Autodesk Inventor part; units mm, degrees
ref_plane "YZ Plane" through (0, 0, 0) normal (1, 0, 0) x (0, 1, 0)
ref_plane "XZ Plane" through (0, 0, 0) normal (0, 1, 0) x (-1, 0, 0)
ref_plane "XY Plane" through (0, 0, 0) normal (0, 0, 1) x (1, 0, 0)
sketch "Sketch1" plane through (0, 0, 0) normal (0, 1, 0) x (-1, 0, 0)
  line L0 (0, 0) -> (762, 0)
  line L1 (762, 0) -> (762, 50.8)
  line L2 (762, 50.8) -> (0, 50.8)
  line L3 (0, 50.8) -> (0, 0)
  dimension "d0" = 762
  dimension "d1" = 50.8
extrude "Extrusion1" add sketch "Sketch1" along normal blind 3.175
sketch "Sketch2" plane through (0, 3.175, 0) normal (0, 1, 0) x (1, 0, 0)
  circle A0 centre (-381, -28.575) radius 4.7625
  line L0 (0, 0) -> (-762, 0)
  line L1 (0, -50.8) -> (0, 0)
  circle A1 centre (-114.3, -12.7) radius 4.7625
  line L2 (-762, -50.8) -> (0, -50.8)
  circle A2 centre (-647.7, -12.7) radius 4.7625
  line L3 (-647.7, 0) -> (-647.7, -50.8) construction
  line L4 (-762, -50.8) -> (0, -50.8) construction
  line L5 (-114.3, -50.8) -> (-114.3, 0) construction
  circle A3 centre (-558.8, -25.4) radius 3.3734
  line L6 (-762, 0) -> (-762, -50.8)
  circle A4 centre (-495.3, -25.4) radius 3.3734
  circle A5 centre (-203.2, -25.4) radius 3.3734
  circle A6 centre (-266.7, -25.4) radius 3.3734
  dimension "d4" = 9.525
  dimension "d5" = 28.575
  dimension "d6" = 381
  dimension "d9" = 9.525
  dimension "d10" = 38.1
  dimension "d12" = 9.525
  dimension "d13" = 38.1
  dimension "d31" = 266.7
  dimension "d32" = 266.7
  dimension "d33" = 6.7469
  dimension "d34" = 203.2
  dimension "d35" = 25.4
  dimension "d36" = 6.7469
  dimension "d37" = 25.4
  dimension "d38" = 266.7
  dimension "d39" = 6.7469
  dimension "d40" = 6.7469
  dimension "d41" = 25.4
  dimension "d42" = 25.4
  dimension "d43" = 203.2
  dimension "d44" = 266.7
extrude "Extrusion2" cut sketch "Sketch2" against normal blind 3.175 contours A0 | A1 | A2 | A3 | A4 | A5 | A6
sketch "Sketch3" plane through (-762, 0, 50.8) normal (0, 0, 1) x (1, 0, 0)
  line L0 (762, 3.175) -> (0, 3.175)
  line L1 (762, 3.175) -> (0, 3.175)
  line L2 (0, 3.175) -> (0, -19.05)
  line L3 (0, -19.05) -> (762, -19.05)
  line L4 (762, -19.05) -> (762, 3.175)
  point P0 (762, 0)
  dimension "d15" = 762
  dimension "d16" = 22.225
extrude "Extrusion3" add sketch "Sketch3" along normal blind 3.175
sketch "Sketch4" plane through (0, 0, 0) normal (0, 0, -1) x (-1, 0, 0)
  line L0 (0, 3.175) -> (762, 3.175)
  line L1 (762, 3.175) -> (762, -19.05)
  line L2 (762, -19.05) -> (0, -19.05)
  line L3 (0, -19.05) -> (0, 3.175)
  dimension "d19" = 762
  dimension "d20" = 22.225
extrude "Extrusion4" add sketch "Sketch4" along normal blind 3.175
sketch "Sketch5" plane through (-762, 0, 53.975) normal (0, 0, 1) x (1, 0, 0)
  line L0 (762, -19.05) -> (0, -19.05)
  line L1 (0, 0) -> (762, 0)
  line L2 (730.25, -19.05) -> (565.15, -19.05)
  line L3 (565.15, -19.05) -> (565.15, 0)
  line L4 (565.15, 0) -> (730.25, 0)
  line L5 (730.25, 0) -> (730.25, -19.05)
  line L6 (762, -19.05) -> (762, 3.175)
  line L7 (488.95, -19.05) -> (273.05, -19.05)
  line L8 (273.05, -19.05) -> (273.05, 0)
  line L9 (273.05, 0) -> (488.95, 0)
  line L10 (488.95, 0) -> (488.95, -19.05)
  line L11 (31.75, -19.05) -> (196.85, -19.05)
  line L12 (196.85, -19.05) -> (196.85, 0)
  line L13 (196.85, 0) -> (31.75, 0)
  line L14 (31.75, 0) -> (31.75, -19.05)
  line L15 (0, 3.175) -> (0, -19.05)
  dimension "d23" = 165.1
  dimension "d24" = 31.75
  dimension "d25" = 215.9
  dimension "d26" = 76.2
  dimension "d27" = 165.1
  dimension "d28" = 31.75
extrude "Extrusion5" cut sketch "Sketch5" against normal blind 57.15 contours L0 L3 L1 L5 | L0 L8 L1 L10 | L0 L14 L1 L12
properties part number "side plate" material "Aluminum 6061"
Can you work these out from the model? Positions are in its coordinate system, mm. A direction names the side the tool comes from. Give positions to 0.01 mm unless a question says otherwise; leave off trailing zeros. Order: outer loops, then holes, each group sorted by start corner. A loop starts at its lowest first (then second) coordinate and runs counter-clockwise, first axis right, second up. Notation, with made-up numbers: M -11.5,39 L -2.5,39 A31 cw -2.5,68 Z; hole C 33.5,-17 d1. An arc over 180 degrees is marked long. One line per item, written item: value.
1) On a 3-axis mill with a long thin cutter (end or side, diameter ignored), from which of +Z, -Z, +X, -X, +Y, -Y can I reach the whole of each face in a straight line? I mean faces 4 (the face through (-746, -9, 50.8)), 5 (the face through (-376, 3.175, 26)). Say none if no direction works.
Answer sheet:
face 4: +X, -X, -Y
face 5: +Z, -Z, +X, -X, +Y
2) For P1, Ø8, axis at x = -266.7, z = 25.4, coming from the -Y side; P2, Ø4, axis at x = -203.2, z = 25.4, coming from the -Y side; P3, Ø1.5, axis at y = 0.5, z = 19, coming from the +X side, each with a flat end and sliding along its axis, tell me the tip position at first contact or that it passes through.
Answer sheet:
P1: stops at y = 0
P2: passes through
P3: stops at x = 0
3) I want a section at C-C, the plane z = 40. List the corners of the cut face in (x, y) for me (3 decimals).
Answer sheet:
outline: M -762,0 L 0,0 L 0,3.175 L -762,3.175 Z
4) Please list where these lines run through material, in increasing order: line 1 along Z through (x, y) = (-515.5, -14.5) (3 decimals); line 2 along Z through (x, y) = (-266.7, 0.8) (3 decimals); line 3 along X through (y, z) = (1.65, 25.4).
Answer sheet:
line 1: z = -3.175 to 0, 50.8 to 53.975
line 2: z = -3.175 to 22.027, 28.773 to 53.975
line 3: x = -762 to -562.17, -555.43 to -498.67, -491.93 to -384.55, -377.45 to -270.07, -263.33 to -206.57, -199.83 to 0
5) I want a section at B-B, the plane x = -400.5. List the corners of the cut face in (y, z) for me (3 decimals), plus the area to 3 significant figures.
Answer sheet:
outline: M 0,-3.175 L 3.175,-3.175 L 3.175,53.975 L 0,53.975 Z
area: 181 mm^2
6) I want a section at A-A, the plane y = -7. Count the separate pieces of the cut face and the enclosed holes in it, plus the area to 3 significant figures.
Answer sheet:
separate pieces: 8
enclosed holes: 0
area: 1,370 mm^2
7) We'd pull the mould along Z, two halves only. Please class faces 1 (the face through (0, 0.2, 27.7)), 2 (the face through (-16, -9, 0)), 3 (the face through (-383, 3, 53.975)): released by +Z, released by -Z, zero draft, split by the parting line, or undercut.
Answer sheet:
face 1: zero draft
face 2: undercut
face 3: released by +Z
